Autodesk Inventor part; units mm, degrees
ref_plane "YZ Plane" through (0, 0, 0) normal (1, 0, 0) x (0, 1, 0)
ref_plane "XZ Plane" through (0, 0, 0) normal (0, 1, 0) x (-1, 0, 0)
ref_plane "XY Plane" through (0, 0, 0) normal (0, 0, 1) x (1, 0, 0)
sketch "Sketch1" plane through (0, 0, 0) normal (0, 1, 0) x (-1, 0, 0)
  line L0 (14, 7.5) -> (-14, 7.5)
  line L1 (-14, 7.5) -> (-14, -7.5)
  line L2 (-14, -7.5) -> (14, -7.5)
  line L3 (14, -7.5) -> (14, 7.5)
  line L4 (14, 7.5) -> (-14, -7.5) construction
  line L5 (-14, 7.5) -> (14, -7.5) construction
  point P0 (0, 0)
  dimension "d0" = 28
  dimension "d1" = 15
extrude "Extrusion1" add sketch "Sketch1" along normal blind 10
sketch "Sketch2" plane through (-14, 0, 7.5) normal (0, 0, 1) x (1, 0, 0)
  line L0 (15.5, 7) -> (40.5, 7)
  line L1 (40.5, 7) -> (40.5, 3)
  line L2 (40.5, 3) -> (15.5, 3)
  line L3 (15.5, 3) -> (15.5, 7)
  line L4 (28, 0) -> (28, 10)
  line L5 (15.5, 7) -> (40.5, 3) construction
  line L6 (40.5, 7) -> (15.5, 3) construction
  point P0 (14, 0)
  point P1 (28, 5)
  dimension "d4" = 25
  dimension "d5" = 4
extrude "Extrusion2" add sketch "Sketch2" along normal blind 3
sketch "Sketch3" plane through (14, 0, -7.5) normal (0, 0, -1) x (-1, 0, 0)
  line L0 (0, 3) -> (0, 7)
  line L1 (0, 5) -> (15, 5)
  line L2 (16.5, 3) -> (13.5, 3)
  line L3 (13.5, 3) -> (13.5, 7)
  line L4 (13.5, 7) -> (16.5, 7)
  line L5 (16.5, 7) -> (16.5, 3)
  line L6 (16.5, 3) -> (13.5, 7) construction
  line L7 (13.5, 3) -> (16.5, 7) construction
  line L8 (15, 3) -> (15, 7)
  point P0 (14, 0)
  dimension "d8" = 15
  dimension "d9" = 3
extrude "Extrusion3" add sketch "Sketch3" along normal blind 5 contours L8 L4 L5 L2
sketch "Sketch4" plane through (-2.5, 3, -7.5) normal (-1, 0, 0) x (0, 0, 1)
  line L0 (-5, 4) -> (-5, 0)
  line L1 (-5, 4) -> (-3, 4)
  line L2 (-3, 4) -> (-3, 0)
  line L3 (-3, 0) -> (-5, 0)
  line L4 (-5, 0) -> (-5, 4)
  point P0 (7.5, -3)
  dimension "d12" = 2
extrude "Extrusion4" add sketch "Sketch4" along normal blind 6
sketch "Sketch5" plane through (-14, 0, -7.5) normal (-1, 0, 0) x (0, 0, 1)
  line L0 (0, 0) -> (0, 10)
  line L1 (0, 5) -> (4, 5)
  line L2 (6, 3) -> (2, 3)
  line L3 (2, 3) -> (2, 7)
  line L4 (2, 7) -> (6, 7)
  line L5 (6, 7) -> (6, 3)
  line L6 (6, 3) -> (2, 7) construction
  line L7 (2, 3) -> (6, 7) construction
  line L8 (4, 3) -> (4, 7)
  line L9 (7.5, 0) -> (7.5, 3)
  line L10 (15, 5) -> (11, 5)
  line L11 (9, 3) -> (13, 3)
  line L12 (13, 3) -> (13, 7)
  line L13 (13, 7) -> (9, 7)
  line L14 (9, 7) -> (9, 3)
  line L15 (9, 3) -> (13, 7) construction
  line L16 (13, 3) -> (9, 7) construction
  line L17 (11, 3) -> (11, 7)
  dimension "d15" = 4
  dimension "d16" = 4
  dimension "d17" = 4
  dimension "d18" = 3
extrude "Extrusion5" add sketch "Sketch5" along normal blind 6 contours L8 L4 L5 L2 | L17 L11 L14 L13
sketch "Sketch7" plane through (0, 0, 0) normal (0, -1, 0) x (1, 0, 0)
  line L0 (14, 7.5) -> (14, -7.5)
  line L1 (-14, -7.5) -> (-14, 7.5)
  line L2 (11, -5) -> (-11, -5)
  line L3 (-11, -5) -> (-11, 5)
  line L4 (-11, 5) -> (11, 5)
  line L5 (11, 5) -> (11, -5)
  line L6 (11, -5) -> (-11, 5) construction
  line L7 (-11, -5) -> (11, 5) construction
  circle A0 centre (-11, 5) radius 1.5
  circle A1 centre (11, -5) radius 1.5
  point P0 (0, 0)
  dimension "d40" = 22
  dimension "d41" = 10
  dimension "d42" = 3
  dimension "d43" = 3
extrude "Extrusion7" cut sketch "Sketch7" against normal blind 15 contours L5 A1 L2 | L2 A1 L5 | A0 L4 L3 | L3 L4 A0
properties part number "FINAL_DE_CARRERA"
Can you work these out from the model? Positions are in its coordinate system, mm. A direction names the side the tool comes from. Give positions to 0.01 mm unless a question says otherwise; leave off trailing zeros. Loops run counter-clockwise (first coordinate to the right, second up) from the corner with the lowest first, then second, coordinate; pieces in that order, holes last. Notation, with made-up numbers: (59, 26) -> (68, 26) arc R34 ccw to (68, 59) -> close; hole circle Ø6 at (-11, 24). An arc over 180 degrees is marked (long way). Use one line per item in the form item = value.
1) If we section it at B-B (z = -5): Please give me the cut outline in (x, y).
Answers:
outline = (-14, 0) -> (9.5, 0) -> (9.5, 10) -> (-14, 10) -> close; (12.5, 0) -> (14, 0) -> (14, 10) -> (12.5, 10) -> close
2) If we section it at D-D (x = 3.5): Please give me the cut outline in (y, z), plus the area to 3 significant figures.
Answers:
outline = (0, -7.5) -> (10, -7.5) -> (10, 7.5) -> (7, 7.5) -> (7, 10.5) -> (3, 10.5) -> (3, 7.5) -> (0, 7.5) -> close
area = 162 mm²
3) Will these pins go through, and if not, where does the flat tip stop? pin 1 (4.5 mm diameter, centred on x = -18, y = 4.5, fed in from -Z); pin 2 (1.5 mm diameter, centred on y = 4.5, z = 9, fed in from -X); pin 3 (2.5 mm diameter, centred on x = 11.5, z = 9.5, fed in from +Y).
Answers:
pin_1 = -3.5
pin_2 = 1.5
pin_3 = 7
4) If we section it at A-A (x = -6.5): Please give me the cut outline in (y, z).
Answers:
outline = (0, -7.5) -> (10, -7.5) -> (10, 7.5) -> (0, 7.5) -> close; (3, -12.5) -> (7, -12.5) -> (7, -10.5) -> (3, -10.5) -> close
5) If we section it at C-C (y = 6.25): Please give me the cut outline in (x, z).
Answers:
outline = (-20, -3.5) -> (-14, -3.5) -> (-14, -7.5) -> (-2.5, -7.5) -> (-2.5, -10.5) -> (-8.5, -10.5) -> (-8.5, -12.5) -> (-1, -12.5) -> (-1, -7.5) -> (14, -7.5) -> (14, 7.5) -> (26.5, 7.5) -> (26.5, 10.5) -> (1.5, 10.5) -> (1.5, 7.5) -> (-14, 7.5) -> (-14, 3.5) -> (-20, 3.5) -> (-20, 1.5) -> (-14, 1.5) -> (-14, -1.5) -> (-20, -1.5) -> close; hole circle Ø3 at (-11, 5); hole circle Ø3 at (11, -5)
6) I need wall thicknesses on line 1 along Z through (x, y) = (11, 4.5); line 2 along X through (y, z) = (3.75, 5); line 3 along Z through (x, y) = (11, 2.5). Which ranges of each line are inside material? Lowest first, please.
Answers:
line_1 = -7.5 to -6.5, -3.5 to 10.5
line_2 = -14 to -12.5, -9.5 to 14
line_3 = -7.5 to -6.5, -3.5 to 7.5
7) For faces 1 (the face through (-17, 5, 1.5)), 2 (the face through (-4, 7, -11)), 3 (the face through (-8.5, 5, -12)), 4 (the face through (-4, 3, -11)), 5 (the face through (-17, 3, 2)), which set-ups out of +Z, -Z, +X, -X, +Y, -Y let a thin tool reach every point of the face, with its end or its side?
Answers:
face_1 = -X, +Y, -Y
face_2 = -Z, +X, -X, +Y
face_3 = -Z, -X, +Y, -Y
face_4 = -Z, +X, -X, -Y
face_5 = +Z, -Z, -X, -Y
8) We'd pull the mould along Z, two halves only. Please class faces 6 (the face through (14, 5, 0)), 7 (the face through (-17, 5, -1.5)), 8 (the face through (14, 5, 10.5)), 9 (the face through (-5, 5, -12.5)): released by +Z, released by -Z, zero draft, split by the parting line, or undercut.
Answers:
face_6 = zero draft
face_7 = undercut
face_8 = released by +Z
face_9 = released by -Z
